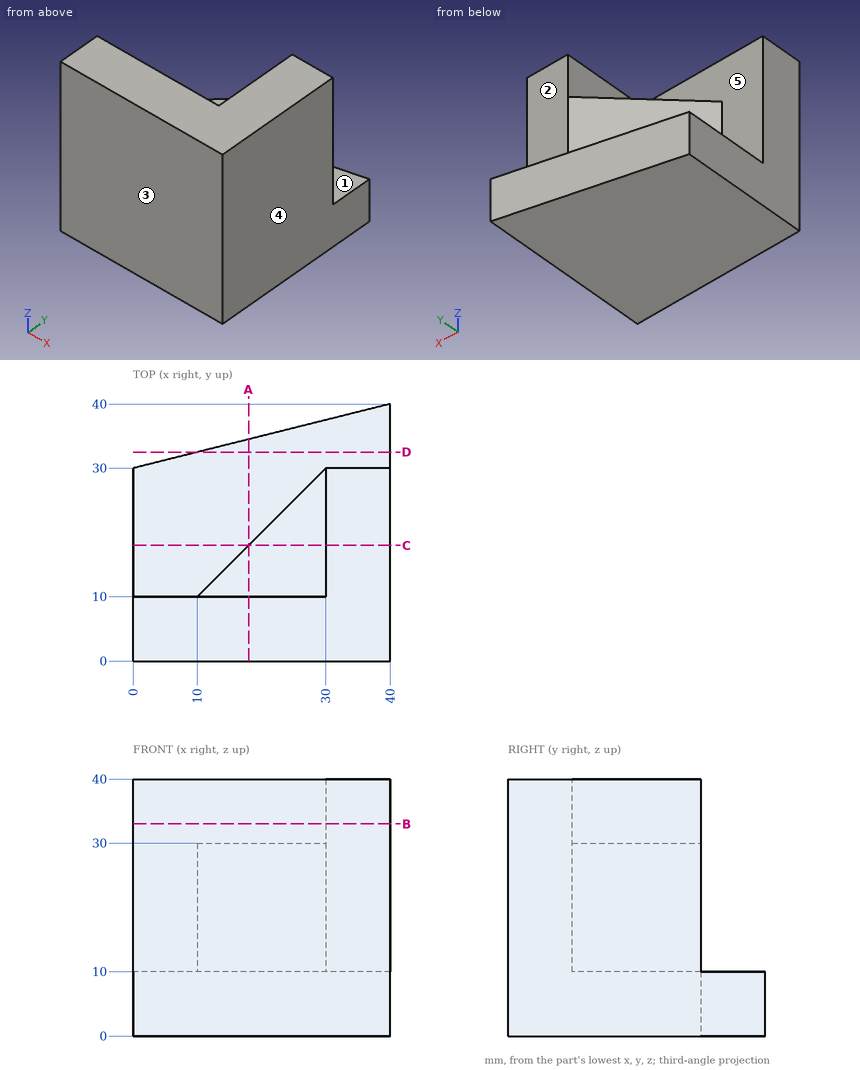
Input: dimensioned drawing with shaded views. Units: mm. Origin: part minimum x, y, z. A direction names the side the tool comes from. Give positions to 0.01 mm unless a question says otherwise; leave off trailing zeros. Order: outer loops, then holes, each group sorted by start corner. A loop starts at its lowest first (then second) coordinate and runs counter-clockwise, first axis right, second up.
(1) Section query D-D (y = 32.5). Return the cut outline in (x, z).
(2) Section query C-C (y = 18). Return the cut outline in (x, z).
(3) Access query for the marked faces 4 and 5. Directions: +Z, -Z, +X, -X, +Y, -Y. A direction counts if a zero-diameter tool reaches every point of the face in a straight line with its end or side. Return the directions, or none.
(4) Section query A-A (x = 18). Return the cut outline in (y, z).
(5) Pull-direction query (Y, two-part tool) for the marked faces 1, 2 and 3; classes: +Y half, -Y half, draft (parallel to the pull), parting line (faces both ways), or undercut.
(6) Section query B-B (z = 33). Return the cut outline in (x, y).
(7) Material intervals for line 1 along X through (y, z) = (24.5, 32); line 2 along Y through (x, z) = (7, 33.5); line 3 along Z through (x, y) = (26, 19), sorted ascending.
(8) Contact query for flat-ended pins moving along their axis: P1, Ø5, axis at y = 19, z = 31, coming from the -X side; P2, Ø6, axis at x = 26, z = 27, coming from the +Y side; P3, Ø8, axis at x = 34, z = 30, coming from the +Y side. Output: stop coordinate, or through.
Outcome:
1. outline: (10, 0) - (40, 0) - (40, 10) - (10, 10) - close
2. outline: (0, 0) - (40, 0) - (40, 40) - (30, 40) - (30, 30) - (18, 30) - (18, 10) - (0, 10) - close
3. face 4: +Z, -Z, +X, +Y, -Y
3. face 5: +Z, -X, +Y
4. outline: (0, 0) - (34.5, 0) - (34.5, 10) - (18, 10) - (18, 30) - (10, 30) - (10, 40) - (0, 40) - close
5. face 1: draft
5. face 2: +Y half
5. face 3: -Y half
6. outline: (0, 0) - (40, 0) - (40, 30) - (30, 30) - (30, 10) - (0, 10) - close
7. line 1: x = 30 to 40
7. line 2: y = 0 to 10
7. line 3: z = 0 to 30
8. P1: stops at x = 16.71
8. P2: stops at y = 29
8. P3: stops at y = 30
